Build history of the part. All positions in model axes, mm. A direction names the side the tool comes from. Give positions to 0.01 mm unless a question says otherwise; leave off trailing zeros. Order: outer loops, then holes, each group sorted by start corner. A loop starts at its lowest first (then second) coordinate and runs counter-clockwise, first axis right, second up. Notation, with made-up numbers: (67.5, 67) -> (97.5, 67) arc R10 cw to (97.5, 80) -> close; hole circle Ø10 at (17.25, 59). An arc over 180 degrees is marked (long way). One line per item, written item: value. Start each with the question number.
(1) Saw through at D-D on x = 107.95. Give the cut face in (y, z) (3 decimals), plus the area to 3 significant figures.
(2) Saw through at A-A on x = 35. Give the cut face in (y, z).
(3) Saw through at C-C on z = -93.98. Give the cut face in (x, y) (3 decimals), plus the area to 3 significant figures.
(4) Saw through at B-B on y = -2.7. Give the cut face in (x, z) (3 decimals).
(5) Probe line 1 (Z direction, x = 67, y = -3.3); line 2 (Z direction, x = 57.15, y = -3.25) (3 decimals); line 3 (X direction, y = -1.35, z = -52.07) (3 decimals). List the from-to ranges inside material, lowest first.
(6) Which spindle directions (+Z, -Z, +X, -X, +Y, -Y) get a long thin tool onto all of the face, cutting with end or side? Do faces 4 (the flat face through (81, -3, -187.96)), 5 (the flat face through (20.32, -3, -18)). Say none if no direction does.
(7) Two-plate mould, pull along X, no slides. Class faces 1 (the flat face through (81, -3, 0)), 2 (the flat face through (165.1, -3, -95)), 3 (the flat face through (20.32, -3, -170)): +X half, -X half, draft (parallel to the pull), parting line (faces both ways), or undercut.
```python
from build123d import *

# Parameters (mm, degrees)
F0_W     = 165.1
F0_H     = 187.96
F1_DEPTH = 5.08
F2_W     = 124.46
F2_H     = 5.08
F3_DEPTH = 25.4
F5_DEPTH = 25.4


with BuildPart() as f1:
    # F0 (on Front) → F1 (new body)
    with BuildSketch(Plane.XZ):
        with Locations((82.55, -93.98)):
            Rectangle(F0_W, F0_H)
    extrude(amount=F1_DEPTH)

    # F2 (on face) → F3 (cut)
    with BuildSketch(Plane.XZ.offset(5.08)):
        with Locations((82.55, -17.78)):
            Rectangle(F2_W, F2_H)
        with Locations((82.55, -170.18)):
            Rectangle(F2_W, F2_H)
    extrude(amount=-F3_DEPTH, mode=Mode.SUBTRACT)

    # F4 (on face) → F5 (cut)
    with BuildSketch(Plane.XZ.offset(5.08)):
        with BuildLine():
            ThreePointArc((111.125, -93.98), (107.95, -90.805), (104.775, -93.98))
            ThreePointArc((104.775, -93.98), (107.95, -97.155), (111.125, -93.98))
        make_face()
        with BuildLine():
            ThreePointArc((60.325, -135.89), (59.395064, -133.644936), (57.15, -132.715))
            ThreePointArc((57.15, -132.715), (54.904936, -138.135064), (60.325, -135.89))
        make_face()
        with BuildLine():
            ThreePointArc((60.325, -52.07), (54.904936, -49.824936), (57.15, -55.245))
            ThreePointArc((57.15, -55.245), (59.395064, -54.315064), (60.325, -52.07))
        make_face()
    extrude(amount=-F5_DEPTH, mode=Mode.SUBTRACT)


solid = f1.part
```
Results below:
1. outline: (-5.08, -187.96) -> (0, -187.96) -> (0, -172.72) -> (-5.08, -172.72) -> close; (-5.08, -167.64) -> (0, -167.64) -> (0, -97.155) -> (-5.08, -97.155) -> close; (-5.08, -90.805) -> (0, -90.805) -> (0, -20.32) -> (-5.08, -20.32) -> close; (-5.08, -15.24) -> (0, -15.24) -> (0, 0) -> (-5.08, 0) -> close
1. area: 871 mm²
2. outline: (-5.08, -187.96) -> (0, -187.96) -> (0, -172.72) -> (-5.08, -172.72) -> close; (-5.08, -167.64) -> (0, -167.64) -> (0, -20.32) -> (-5.08, -20.32) -> close; (-5.08, -15.24) -> (0, -15.24) -> (0, 0) -> (-5.08, 0) -> close
3. outline: (0, -5.08) -> (104.775, -5.08) -> (104.775, 0) -> (0, 0) -> close; (111.125, -5.08) -> (165.1, -5.08) -> (165.1, 0) -> (111.125, 0) -> close
3. area: 806 mm²
4. outline: (0, -187.96) -> (165.1, -187.96) -> (165.1, 0) -> (0, 0) -> close; hole (20.32, -172.72) -> (144.78, -172.72) -> (144.78, -167.64) -> (20.32, -167.64) -> close; hole (20.32, -20.32) -> (144.78, -20.32) -> (144.78, -15.24) -> (20.32, -15.24) -> close; hole circle Ø6.35 at (57.15, -135.89); hole circle Ø6.35 at (57.15, -52.07); hole circle Ø6.35 at (107.95, -93.98)
5. line 1: z = -187.96 to -172.72, -167.64 to -20.32, -15.24 to 0
5. line 2: z = -187.96 to -172.72, -167.64 to -139.065, -132.715 to -55.245, -48.895 to -20.32, -15.24 to 0
5. line 3: x = 0 to 53.975, 60.325 to 165.1
6. face 4: -Z, +X, -X, +Y, -Y
6. face 5: +Y, -Y
7. face 1: draft
7. face 2: +X half
7. face 3: undercut
